from build123d import *

# Parameters (mm, degrees)
ESQUISSE1_W             = 197.55
ESQUISSE1_H             = 40
BOSS_EXTRU_1_DEPTH      = 82
ESQUISSE2_W             = 177.55
ESQUISSE2_H             = 78
ENL_V_MAT_EXTRU_1_DEPTH = 38
ENL_V_MAT_EXTRU_4_DEPTH = 82
BOSS_EXTRU_6_DEPTH      = 78.5
ESQUISSE8_W             = 48
ESQUISSE8_H             = 16.041036462
ENL_V_MAT_EXTRU_5_DEPTH = 26.4
ESQUISSE9_W             = 2.5
ESQUISSE9_H             = 12.2
ENL_V_MAT_EXTRU_6_DEPTH = 26.4
ESQUISSE10_W            = 2.5
ESQUISSE10_H            = 12
ENL_V_MAT_EXTRU_7_DEPTH = 26.4
ENL_V_MAT_EXTRU_9_DEPTH = 82


with BuildPart() as part:
    # Esquisse1 → Boss.-Extru.1 (new body)
    with BuildSketch(Plane.XY):
        with Locations((-98.775, 20)):
            Rectangle(ESQUISSE1_W, ESQUISSE1_H)
    extrude(amount=BOSS_EXTRU_1_DEPTH)

    # Esquisse2 → Enlèv. mat.-Extru.1 (cut)
    with BuildSketch(Plane(origin=(0, 40, 0), x_dir=(1, 0, 0), z_dir=(0, 1, 0))):
        with Locations((-98.775, -41)):
            Rectangle(ESQUISSE2_W, ESQUISSE2_H)
    extrude(amount=-ENL_V_MAT_EXTRU_1_DEPTH, mode=Mode.SUBTRACT)

    # Esquisse3 → Enlèv. mat.-Extru.4 (cut)
    with BuildSketch(Plane.XY):
        Polygon((-197.55, 40), (-189.55, 0), (-197.55, 0), align=None)
        Polygon((0, 40), (-8, 0), (0, 0), align=None)
    extrude(amount=ENL_V_MAT_EXTRU_4_DEPTH, mode=Mode.SUBTRACT)

    # Esquisse6 → Boss.-Extru.6 (add)
    with BuildSketch(Plane.XY.offset(2)):
        Polygon((-175.55, 12.914570305), (-175.55, 0.914570305), (-177.55, 0.914570305), (-177.55, 13.90441537), (-155.74, 30.541036462), (-155.74, 14.5), (-157.74, 14.5), (-157.74, 26.5), align=None)
    extrude(amount=BOSS_EXTRU_6_DEPTH)

    # Esquisse8 → Enlèv. mat.-Extru.5 (cut)
    with BuildSketch(Plane(origin=(-155.74, 0, 0), x_dir=(0, 0, -1), z_dir=(1, 0, 0))):
        with Locations((-41, 22.520518231)):
            Rectangle(ESQUISSE8_W, ESQUISSE8_H)
    extrude(amount=-ENL_V_MAT_EXTRU_5_DEPTH, mode=Mode.SUBTRACT)

    # Esquisse9 → Enlèv. mat.-Extru.6 (cut)
    with BuildSketch(Plane(origin=(-155.74, 0, 0), x_dir=(0, 0, -1), z_dir=(1, 0, 0))):
        with Locations((-74.75, 20.6)):
            Rectangle(ESQUISSE9_W, ESQUISSE9_H)
    extrude(amount=-ENL_V_MAT_EXTRU_6_DEPTH, mode=Mode.SUBTRACT)

    # Esquisse10 → Enlèv. mat.-Extru.7 (cut)
    with BuildSketch(Plane(origin=(-155.74, 0, 0), x_dir=(0, 0, -1), z_dir=(1, 0, 0))):
        with Locations((-7.25, 20.5)):
            Rectangle(ESQUISSE10_W, ESQUISSE10_H)
    extrude(amount=-ENL_V_MAT_EXTRU_7_DEPTH, mode=Mode.SUBTRACT)

    # Esquisse11 → Enlèv. mat.-Extru.9 (cut)
    with BuildSketch(Plane(origin=(0, 0, 0), x_dir=(-1, 0, 0), z_dir=(0, 0, -1))):
        Polygon((175.55, 12.914570305), (160.55, 24.356538044), (160.55, 12.356538044), (175.55, 12.356538044), align=None)
    extrude(amount=-ENL_V_MAT_EXTRU_9_DEPTH, mode=Mode.SUBTRACT)


solid = part.part
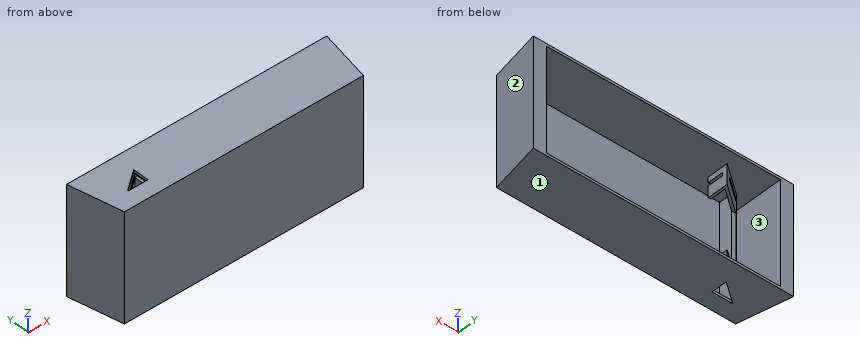
Model file for the job. Use its own axes, mm. Face numbers are marked on the shaded views. Coordinates: 2 decimals unless noted, no trailing zeros. Order: outer loops, then holes, each group sorted by start corner. A loop starts at its lowest first (then second) coordinate and runs counter-clockwise, first axis right, second up. Notation, with made-up numbers: M -28,2.5 L 31,2.5 A23 cw 31,40.5 Z; hole C 28,7.25 d4. An arc over 180 degrees is marked long. Return JSON: item names as keys, results as strings.
1. Flat gauge pins, fed straight in: pin 1 (2 mm diameter, centred on y = 9, z = 35.5, fed in from +X); pin 2 (16.5 mm diameter, centred on y = 19, z = 69.5, fed in from +X); pin 3 (1 mm diameter, centred on x = -174, z = 61.5, fed in from +Y). Where does each tip first touch, or does it go through?
Ans:
{"pin 1": "x = -6", "pin 2": "x = -2.55", "pin 3": "y = 14.5"}
2. Saw through at A-A (y = 35). Give the cut face in (x, z), and give its area (3 significant figures).
Ans:
{"outline": "M -196.55,0 L -1,0 L -1,82 L -196.55,82 Z; hole M -187.55,2 L -10,2 L -10,80 L -187.55,80 Z", "area": "2,190 mm^2"}
3. Saw through at B-B (x = -15). Give the cut face in (y, z), and give its area (3 significant figures).
Ans:
{"outline": "M 0,0 L 40,0 L 40,2 L 2,2 L 2,80 L 40,80 L 40,82 L 0,82 Z", "area": "316 mm^2"}
4. Saw through at D-D (z = 39). Give the cut face in (x, y).
Ans:
{"outline": "M -197.55,40 L -189.55,0 L -8,0 L 0,40 L -10,40 L -10,2 L -175.55,2 L -175.55,12.91 L -173.47,14.5 L -176.77,14.5 L -177.55,13.9 L -177.55,2 L -187.55,2 L -187.55,40 Z"}
5. Saw through at C-C (z = 11). Give the cut face in (x, y), and give its area (3 significant figures).
Ans:
{"outline": "M -197.55,40 L -189.55,0 L -8,0 L 0,40 L -10,40 L -10,2 L -175.55,2 L -175.55,12.91 L -157.74,26.5 L -157.74,14.5 L -155.74,14.5 L -155.74,30.54 L -177.55,13.9 L -177.55,2 L -187.55,2 L -187.55,40 Z", "area": "936 mm^2"}
6. Pull direction Z, two halves, no side cores. Call the marked faces 1, 2 and 3: +Z half, -Z half, draft (parallel to the pull), parting line (faces both ways), or undercut.
Ans:
{"face 1": "-Z half", "face 2": "draft", "face 3": "undercut"}
7. Drill centre lines: probe 1 along Z at (x, y) = (-106.5, 4); probe 2 along X at (y, z) = (11, 30); probe 3 along X at (y, z) = (18, 15). Where is each one in solid material? Low to high.
Ans:
{"probe 1": "0 to 2, 80 to 82", "probe 2": "-191.75 to -187.55, -177.55 to -175.55, -10 to -5.8", "probe 3": "-193.15 to -187.55, -172.18 to -168.88, -157.74 to -155.74, -10 to -4.4"}
